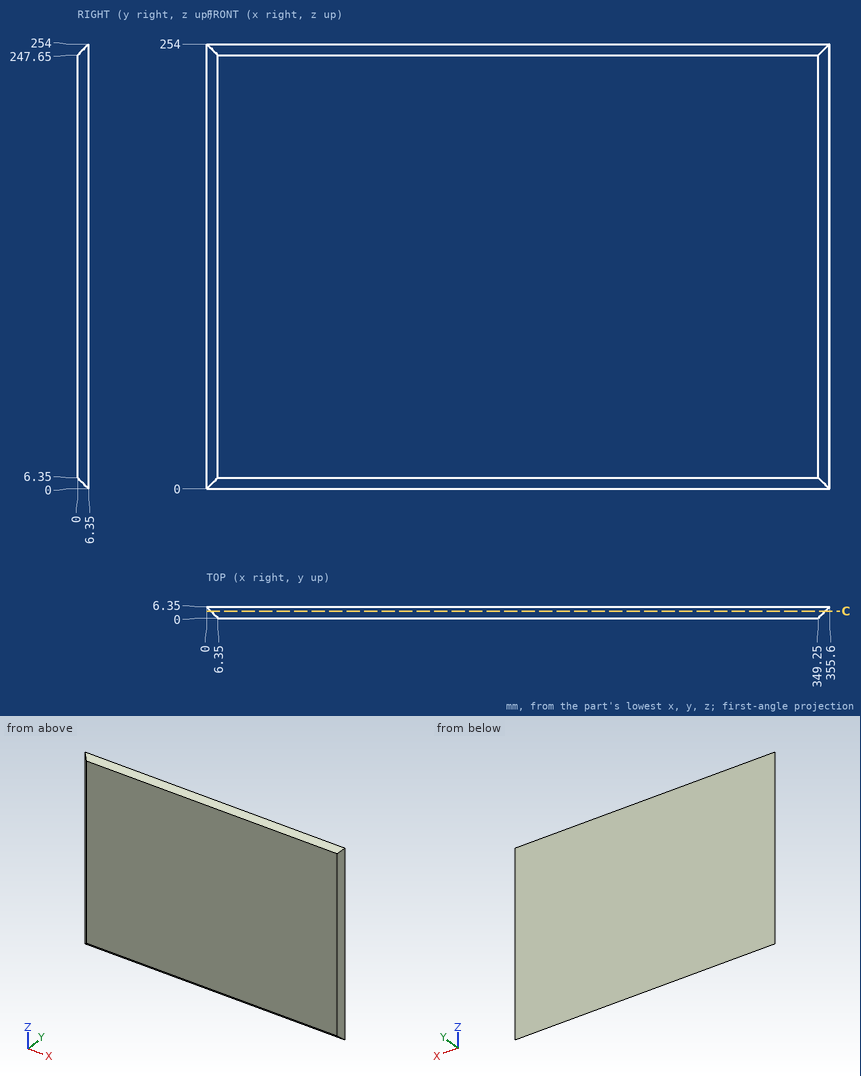
Verification items for this drawing (mm, ordinates from the low corner). Coordinates: 2 decimals unless noted, no trailing zeros. Loops run counter-clockwise (first coordinate to the right, second up) from the corner with the lowest first, then second, coordinate; pieces in that order, holes last. Notation, with made-up numbers: (-30, 37.5) -> (27, 37.5) arc R6 ccw to (27, 46.5) -> close; hole circle Ø1 at (84, 49.25). An arc over 180 degrees is marked (long way). Put each result on its own line as item: value.
1. Thickness scan on line 1 (Z direction, x = 304.5, y = 2.25); line 2 (X direction, y = 3, z = 137); line 3 (X direction, y = 5, z = 182.5). Record the ranges inside material, lowest first.
Result set:
line 1: z = 4.1 to 249.9
line 2: x = 3.35 to 352.25
line 3: x = 1.35 to 354.25
2. Section check C-C, the plane y = 4. Record the boundary of the cut face in (x, z), then the cut area to 3 significant figures.
Result set:
outline: (2.35, 2.35) -> (353.25, 2.35) -> (353.25, 251.65) -> (2.35, 251.65) -> close
area: 87,500 mm^2
3. Gauge pin test, flat end, axial feed: P1, Ø2, axis at x = 292.5, y = 4, coming from the +Z side. Record the tip position at first contact, or that the pin passes through.
Result set:
P1: stops at z = 252.65
